Geometry check sheet. Reference: the model listing, model coordinates, mm. Face numbers are marked on the shaded views. Give positions to 0.01 mm unless a question says otherwise; leave off trailing zeros. Order: outer loops, then holes, each group sorted by start corner. A loop starts at its lowest first (then second) coordinate and runs counter-clockwise, first axis right, second up. Notation, with made-up numbers: M 43,-29 L 78,-29 A17 ccw 78,-18 Z; hole C -12,32.25 d1. An arc over 180 degrees is marked long. Answer as CSV lines item,"result".
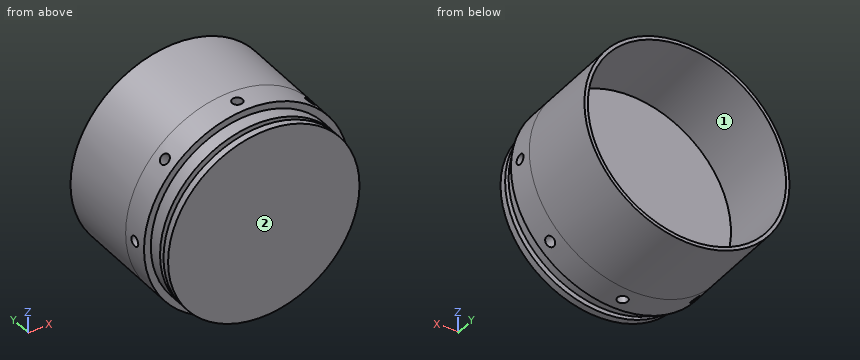
Autodesk Inventor part; units mm, degrees
ref_plane "YZ Plane" through (0, 0, 0) normal (1, 0, 0) x (0, 1, 0)
ref_plane "XZ Plane" through (0, 0, 0) normal (0, 1, 0) x (-1, 0, 0)
ref_plane "XY Plane" through (0, 0, 0) normal (0, 0, 1) x (1, 0, 0)
sketch "Sketch1" plane through (0, 0, 0) normal (0, 0, 1) x (1, 0, 0)
  line L0 (0, 0) -> (-88.9, 0)
  line L1 (-88.9, 0) -> (-88.9, -12.7)
  line L2 (-88.9, -12.7) -> (-82.55, -12.7)
  line L3 (-82.55, -12.7) -> (-82.55, -17.4752)
  line L4 (-82.55, -17.4752) -> (-88.9, -17.4752)
  line L5 (-88.9, -17.4752) -> (-88.9, -23.8252)
  line L6 (-88.9, -23.8252) -> (0, -23.8252)
  line L7 (0, 0) -> (0, 146.0976) construction
  line L8 (-88.9, 0) -> (-95.25, 0)
  line L9 (-95.25, 0) -> (-95.25, 25.4)
  line L10 (-95.25, 25.4) -> (0, 25.4)
  line L11 (0, 25.4) -> (0, -23.8252)
  dimension "d1" = 4.7752
  dimension "d2" = 88.9
  dimension "d3" = 0
  dimension "d5" = 95.25
  dimension "d6" = 6.35
  dimension "d7" = 12.7
  dimension "d8" = 25.4
  dimension "d13" = 6.35
  dimension "d21" = 6.35
revolve "Revolution1" add sketch "Sketch1" angle 360 about axis through (0, 0, 0) along (0, 1, 0)
sketch "Sketch2" plane through (0, 25.4, 0) normal (0, 1, 0) x (1, 0, 0)
  circle A0 centre (0, 0) radius 95.25
  circle A1 centre (0, 0) radius 92.075
  dimension "d9" = 190.5
  dimension "d10" = 184.15
extrude "Extrusion1" add sketch "Sketch2" along normal blind 76.2
sketch "Sketch3" plane through (0, 0, 0) normal (1, 0, 0) x (0, 1, 0)
  circle A0 centre (12.7, 0) radius 4.7625
  line L0 (0, -88.9) -> (0, 88.9)
  point P0 (0, 0)
  dimension "d14" = 12.7
  dimension "d15" = 9.525
extrude "Extrusion2" cut sketch "Sketch3" against normal blind 127
pattern_circular "Circular Pattern1" count 8 over 360 about axis through (0, -10, 0) along (0, 1, 0) of "Extrusion2"
properties part number "ForwardBulkHead"
(1) Material ranges on line 1 (Y direction, x = 29.5, z = 0); line 2 (Z direction, x = 0, y = 78) (3 decimals); line 3 (Y direction, x = 36.5, z = -21.5), recorded low to high.
The answers:
line 1,"y = -23.83 to 7.94, 17.46 to 25.4"
line 2,"z = -95.25 to -92.075, 92.075 to 95.25"
line 3,"y = -23.83 to 25.4"
(2) Gauge pin test, flat ends, axial feed: P1, Ø1, axis at x = -10, y = 7, coming from the -Z side; P2, Ø3, axis at y = 4, z = 57, coming from the -X side; P3, Ø2, axis at x = 35.5, z = 47, coming from the +Y side. Record the tip position at first contact, or that the pin passes through.
The answers:
P1,"stops at z = -94.78"
P2,"stops at x = -77.41"
P3,"stops at y = 25.4"
(3) Draft check along X on the marked faces 1 and 2. Enter one of: +X half, -X half, draft (parallel to the pull), parting line (faces both ways), or undercut.
The answers:
face 1,"undercut"
face 2,"draft"
(4) Section check B-B on z = -74. Enter the section's corners in (x, y) (1 decimal).
The answers:
outline,"M -60,0 L -49.3,0 L -49.3,-12.7 L -36.6,-12.7 L -36.6,-17.5 L -49.3,-17.5 L -49.3,-23.8 L 49.3,-23.8 L 49.3,-17.5 L 36.6,-17.5 L 36.6,-12.7 L 49.3,-12.7 L 49.3,0 L 60,0 L 60,101.6 L 54.8,101.6 L 54.8,25.4 L -54.8,25.4 L -54.8,101.6 L -60,101.6 Z; hole C 0,12.7 d9.5"
(5) Section check A-A on y = 12.7. Enter the section's corners in (x, z), then the cut area to 3 significant figures.
The answers:
outline,"M -95.13,-4.76 A95.25 ccw -70.64,-63.9 L -11.5,-4.76 Z; M -95.13,4.76 L -11.5,4.76 L -70.64,63.9 A95.25 ccw Z; M -63.9,-70.64 A95.25 ccw -4.76,-95.13 L -4.76,-11.5 Z; M -63.9,70.64 L -4.76,11.5 L -4.76,95.13 A95.25 ccw Z; M 4.76,-95.13 A95.25 ccw 63.9,-70.64 L 4.76,-11.5 Z; M 4.76,11.5 L 63.9,70.64 A95.25 ccw 4.76,95.13 Z; M 11.5,-4.76 L 70.64,-63.9 A95.25 ccw 95.13,-4.76 Z; M 11.5,4.76 L 95.13,4.76 A95.25 ccw 70.64,63.9 Z"
area,"21,700 mm2"
(6) Section check C-C on y = 92. Enter the section's corners in (x, z) (3 decimals).
The answers:
outline,"C 0,0 d190.5; hole C 0,0 d184.15"
(7) Section check D-D on x = 49.5. State how many separate pieces and enclosed holes the cut face has, then the cut area to 3 significant figures.
The answers:
separate pieces,"1"
enclosed holes,"3"
area,"7,880 mm2"
